CAD build for the part. Positions are in the model's coordinates, mm. Face numbers are marked on the shaded views. A direction names the side the tool comes from. Coordinates: 2 decimals unless noted, no trailing zeros. Loops run counter-clockwise (first coordinate to the right, second up) from the corner with the lowest first, then second, coordinate; pieces in that order, holes last. Notation, with made-up numbers: (81.25, 38.25) -> (130.25, 38.25) arc R16 ccw to (130.25, 66.25) -> close; hole circle Ø11 at (57, -38.75). An arc over 180 degrees is marked (long way). Write each question's results on one line, items separated by ' | '.
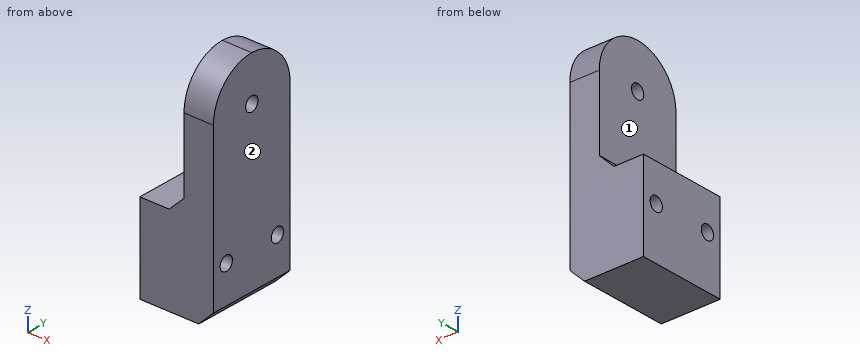
Solid Edge part; units mm, degrees
sketch "Sketch1" plane through (0, 0, 0) normal (0, -1, 0) x (1, 0, 0)
  line L0 (0, 0) -> (0, 30)
  line L1 (0, 30) -> (15, 30)
  line L2 (15, 30) -> (15, 75)
  line L3 (15, 75) -> (25, 75)
  line L4 (25, 75) -> (25, 0)
  line L5 (25, 0) -> (0, 0)
  dimension "D1" = 25
  dimension "D2" = 25
extrude "Protrusion1" add sketch "Sketch1" along normal mid plane 30
fillet "Round_1" radius 15 2 edges at (20, -15, 75) (20, 15, 75)
chamfer "Chamfer_1" distance 5 angle 45 2 edges at (25, 0, 0) (15, 0, 30)
hole "Hole_1" at (25, -10, 17.5) direction (-1, 0, 0) diameter 4.8 end up to next
hole "Hole1" at (25, 10, 17.5) direction (-1, 0, 0) diameter 4.8 end up to next
hole "Hole_3" at (25, 0, 60) direction (-1, 0, 0) diameter 4.8 end up to next
properties material "Polyethylene, low density"
Q1. Wall check: L1, parallel to Y at x = 8.25, z = 17.5; L2, parallel to Z at x = 8, y = 10; L3, parallel to Y at x = 1.75, z = 18.5. Give the ranges that are in metal, low to high. Write a range as from..to.
Results are:
L1: -15..-12.4, -7.6..7.6, 12.4..15 | L2: 0..15.1, 19.9..30 | L3: -15..-12.18, -7.82..7.82, 12.18..15
Q2. Cut at A-A on z = 17.5. Write the cut outline in (x, y), and give its area (3 significant figures).
Results are:
outline: (0, -15) -> (25, -15) -> (25, -12.4) -> (0, -12.4) -> close; (0, -7.6) -> (25, -7.6) -> (25, 7.6) -> (0, 7.6) -> close; (0, 12.4) -> (25, 12.4) -> (25, 15) -> (0, 15) -> close | area: 510 mm^2
Q3. Cut at D-D on x = 8.25. Write the cut outline in (y, z), and give its area (3 significant figures).
Results are:
outline: (-15, 0) -> (15, 0) -> (15, 30) -> (-15, 30) -> close; hole circle Ø4.8 at (-10, 17.5); hole circle Ø4.8 at (10, 17.5) | area: 864 mm^2
Q4. Drop flat-ended pins along their axis: pin 1 (4 mm diameter, centred on x = 9, y = -2.5, fed in from +Z); pin 2 (5 mm diameter, centred on x = 6, y = -4.5, fed in from +Z); pin 3 (7.5 mm diameter, centred on y = 0, z = 60, fed in from -X). Give the stop position or say it passes through.
Results are:
pin 1: z = 31 | pin 2: z = 30 | pin 3: x = 15
Q5. Cut at C-C on y = -10. Write the cut outline in (x, z).
Results are:
outline: (0, 0) -> (20, 0) -> (25, 5) -> (25, 15.1) -> (0, 15.1) -> close; (0, 19.9) -> (25, 19.9) -> (25, 71.18) -> (15, 71.18) -> (15, 35) -> (10, 30) -> (0, 30) -> close
Q6. Which spindle directions (+Z, -Z, +X, -X, +Y, -Y) get a long thin tool onto all of the face, cutting with end or side? Do the marked faces 1 and 2. Say none if no direction does.
Results are:
face 1: +Z, -X, +Y, -Y | face 2: +Z, -Z, +X, +Y, -Y
Q7. Cut at B-B on x = 18.5. Give the number of separate pieces and of enclosed holes in the cut face, and give its area (3 significant figures).
Results are:
separate pieces: 1 | enclosed holes: 3 | area: 2,100 mm^2
